Can you work these out from the model? Positions are in its coordinate system, mm. A direction names the side the tool comes from. Round coordinates to 2 decimals unless told otherwise and drop trailing zeros. Loops run counter-clockwise (first coordinate to the right, second up) from the corner with the lowest first, then second, coordinate; pieces in that order, holes last. Notation, with made-up numbers: M -2.75,17.5 L 28.25,17.5 A18 cw 28.25,42.5 Z; hole C 49.5,-19.5 d10. An arc over 180 degrees is marked long. Return JSON: item names as keys, results as strings.
```python
from build123d import *

# Parameters (mm, degrees)
SKETCH1_W           = 150
SKETCH1_H           = 150
BOSS_EXTRUDE1_DEPTH = 3
CUT_EXTRUDE1_DEPTH  = 264.0332057
SKETCH4_R           = 2.5
CUT_EXTRUDE2_DEPTH  = 3
SKETCH5_R           = 2
CUT_EXTRUDE3_DEPTH  = 10


with BuildPart() as part:
    # Sketch1 → Boss-Extrude1 (new body)
    with BuildSketch(Plane.XY):
        with Locations((146.896551724, 66.206896552)):
            Rectangle(SKETCH1_W, SKETCH1_H)
    extrude(amount=BOSS_EXTRUDE1_DEPTH)

    # Sketch2 → Cut-Extrude1 (cut, through all)
    with BuildSketch(Plane.XY.offset(3)):
        with BuildLine():
            ThreePointArc((188.163122783, 113.13032186), (146.896551724, 128.694797217), (105.629980666, 113.13032186))
            Line((105.629980666, 113.13032186), (112.718359737, 106.041942789))
            ThreePointArc((112.718359737, 106.041942789), (146.896551724, 118.694797217), (181.074743712, 106.041942789))
            Line((181.074743712, 106.041942789), (188.163122783, 113.13032186))
        make_face()
        with BuildLine():
            Line((107.061505487, 100.385088539), (99.973126416, 107.47346761))
            ThreePointArc((99.973126416, 107.47346761), (84.408651059, 66.206896552), (99.973126416, 24.940325493))
            Line((99.973126416, 24.940325493), (107.061505487, 32.028704564))
            ThreePointArc((107.061505487, 32.028704564), (94.408651059, 66.206896552), (107.061505487, 100.385088539))
        make_face()
        with BuildLine():
            ThreePointArc((209.384452389, 66.206896552), (205.363995952, 88.259009716), (193.819977032, 107.47346761))
            Line((193.819977032, 107.47346761), (186.731597961, 100.385088539))
            ThreePointArc((186.731597961, 100.385088539), (196.119705149, 84.429434333), (199.384452389, 66.206896552))
            ThreePointArc((199.384452389, 66.206896552), (196.119705149, 47.984358771), (186.731597961, 32.028704564))
            Line((186.731597961, 32.028704564), (193.819977032, 24.940325493))
            ThreePointArc((193.819977032, 24.940325493), (205.363995952, 44.154783387), (209.384452389, 66.206896552))
        make_face()
        with BuildLine():
            Line((112.718359737, 26.371850315), (105.629980666, 19.283471244))
            ThreePointArc((105.629980666, 19.283471244), (146.896551724, 3.718995886), (188.163122783, 19.283471244))
            Line((188.163122783, 19.283471244), (181.074743712, 26.371850315))
            ThreePointArc((181.074743712, 26.371850315), (146.896551724, 13.718995886), (112.718359737, 26.371850315))
        make_face()
        with BuildLine():
            ThreePointArc((150.896551724, 23.907703853), (176.940034403, 36.163413873), (189.195744423, 62.206896552))
            Line((189.195744423, 62.206896552), (179.137266506, 62.206896552))
            ThreePointArc((179.137266506, 62.206896552), (169.868966591, 43.234481685), (150.896551724, 33.96618177))
            Line((150.896551724, 33.96618177), (150.896551724, 23.907703853))
        make_face()
        with BuildLine():
            Line((114.655836942, 62.206896552), (104.597359026, 62.206896552))
            ThreePointArc((104.597359026, 62.206896552), (116.853069045, 36.163413873), (142.896551724, 23.907703853))
            Line((142.896551724, 23.907703853), (142.896551724, 33.96618177))
            ThreePointArc((142.896551724, 33.96618177), (123.924136857, 43.234481685), (114.655836942, 62.206896552))
        make_face()
        with BuildLine():
            Line((142.896551724, 98.447611333), (142.896551724, 108.50608925))
            ThreePointArc((142.896551724, 108.50608925), (116.853069045, 96.250379231), (104.597359026, 70.206896552))
            Line((104.597359026, 70.206896552), (114.655836942, 70.206896552))
            ThreePointArc((114.655836942, 70.206896552), (123.924136857, 89.179311419), (142.896551724, 98.447611333))
        make_face()
        with BuildLine():
            ThreePointArc((189.195744423, 70.206896552), (176.940034403, 96.250379231), (150.896551724, 108.50608925))
            Line((150.896551724, 108.50608925), (150.896551724, 98.447611333))
            ThreePointArc((150.896551724, 98.447611333), (169.868966591, 89.179311419), (179.137266506, 70.206896552))
            Line((179.137266506, 70.206896552), (189.195744423, 70.206896552))
        make_face()
        with BuildLine():
            Line((165.372753073, 79.026243651), (158.090015102, 71.74350568))
            ThreePointArc((158.090015102, 71.74350568), (159.056537781, 69.049853135), (159.384452389, 66.206896552))
            ThreePointArc((159.384452389, 66.206896552), (159.166880972, 63.885973637), (158.521748029, 61.645923641))
            Line((158.521748029, 61.645923641), (165.932760465, 54.234911206))
            ThreePointArc((165.932760465, 54.234911206), (168.504305512, 59.977076926), (169.384452389, 66.206896552))
            ThreePointArc((169.384452389, 66.206896552), (168.358106385, 72.923096956), (165.372753073, 79.026243651))
        make_face()
        with BuildLine():
            Line((134.077204625, 84.6830979), (141.359942596, 77.400359929))
            ThreePointArc((141.359942596, 77.400359929), (146.896551724, 78.694797217), (152.433160852, 77.400359929))
            Line((152.433160852, 77.400359929), (159.715898823, 84.6830979))
            ThreePointArc((159.715898823, 84.6830979), (146.896551724, 88.694797217), (134.077204625, 84.6830979))
        make_face()
        with BuildLine():
            ThreePointArc((135.703088346, 60.670287424), (134.408651059, 66.206896552), (135.703088346, 71.74350568))
            Line((135.703088346, 71.74350568), (128.420350375, 79.026243651))
            ThreePointArc((128.420350375, 79.026243651), (124.408651059, 66.206896552), (128.420350375, 53.387549452))
            Line((128.420350375, 53.387549452), (135.703088346, 60.670287424))
        make_face()
        with BuildLine():
            ThreePointArc((152.433160852, 55.013433174), (146.896551724, 53.718995886), (141.359942596, 55.013433174))
            Line((141.359942596, 55.013433174), (134.077204625, 47.730695203))
            ThreePointArc((134.077204625, 47.730695203), (146.896551724, 43.718995886), (159.715898823, 47.730695203))
            Line((159.715898823, 47.730695203), (152.433160852, 55.013433174))
        make_face()
    extrude(amount=-CUT_EXTRUDE1_DEPTH, mode=Mode.SUBTRACT)

    # Sketch4 → Cut-Extrude2 (cut)
    with BuildSketch(Plane.XY.offset(3)):
        with Locations((81.896551724, 131.206896552)):
            Circle(SKETCH4_R)
        with Locations((211.896551724, 131.206896552)):
            Circle(SKETCH4_R)
        with Locations((211.896551724, 1.206896552)):
            Circle(SKETCH4_R)
        with Locations((81.896551724, 1.206896552)):
            Circle(SKETCH4_R)
    extrude(amount=-CUT_EXTRUDE2_DEPTH, mode=Mode.SUBTRACT)

    # Sketch5 → Cut-Extrude3 (cut)
    with BuildSketch(Plane.XY.offset(3)):
        with Locations((146.896551724, 66.206896552)):
            Circle(SKETCH5_R)
    extrude(amount=-CUT_EXTRUDE3_DEPTH, mode=Mode.SUBTRACT)


solid = part.part
```
Q1. Suppose I cut it at C-C, the plane x = 176.5. Please give me the cut outline in (y, z).
Results:
{"outline": "M -8.79,0 L 11.18,0 L 11.18,3 L -8.79,3 Z; M 22.86,0 L 35.73,0 L 35.73,3 L 22.86,3 Z; M 52.82,0 L 79.59,0 L 79.59,3 L 52.82,3 Z; M 96.68,0 L 109.55,0 L 109.55,3 L 96.68,3 Z; M 121.24,0 L 141.21,0 L 141.21,3 L 121.24,3 Z"}
Q2. Suppose I cut it at A-A, the plane x = 87.5. Please give me the cut outline in (y, z), plus the area to 3 significant figures.
Results:
{"outline": "M -8.79,0 L 46.8,0 L 46.8,3 L -8.79,3 Z; M 85.62,0 L 141.21,0 L 141.21,3 L 85.62,3 Z", "area": "334 mm2"}
Q3. Suppose I cut it at D-D, the plane x = 207. Please give me the cut outline in (y, z).
Results:
{"outline": "M -8.79,0 L 49.11,0 L 49.11,3 L -8.79,3 Z; M 83.3,0 L 141.21,0 L 141.21,3 L 83.3,3 Z"}
Q4. On a 3-axis mill with a long thin cutter (end or side, diameter ignored), from which of +Z, -Z, +X, -X, +Y, -Y can I reach the whole of each face in a straight line? I mean faces 1 (the flat face through (184.669, 22.778, 1.521)), 2 (the flat face through (163, 51, 3)). Say none if no direction works.
Results:
{"face 1": "+Z, -Z", "face 2": "+Z, +X, -X, +Y, -Y"}
Q5. Suppose I cut it at B-B, the plane y = 36. Please give me the cut outline in (x, z).
Results:
{"outline": "M 71.9,0 L 92.19,0 L 92.19,3 L 71.9,3 Z; M 103.97,0 L 117.02,0 L 117.02,3 L 103.97,3 Z; M 134.94,0 L 158.86,0 L 158.86,3 L 134.94,3 Z; M 176.78,0 L 189.82,0 L 189.82,3 L 176.78,3 Z; M 201.6,0 L 221.9,0 L 221.9,3 L 201.6,3 Z"}
Q6. Thinking about a two-plate mould opening in X: for faces 3 (the flat face through (163, 51, 0)), 4 (the cylindrical face through (169.655, 89.391, 1.521)), 5 (the cylindrical face through (123.712, 88.965, 1.521)), which applies, pulls with the +X half, pulls with the -X half, needs draft (parallel to the pull), parting line crosses it, or undercut?
Results:
{"face 3": "needs draft", "face 4": "undercut", "face 5": "undercut"}
Q7. If I drill on line 1 along X through (y, z) = (99.5, 2.1); line 2 along X through (y, z) = (50, 2.2); line 3 along Y through (x, z) = (164, 0.6), over which ranges is the centre line in solid material (lowest first)?
Results:
{"line 1": "x = 71.9 to 94.02, 106.32 to 120.5, 142.9 to 150.9, 173.29 to 187.47, 199.78 to 221.9", "line 2": "x = 71.9 to 86.55, 96.97 to 107.62, 118.74 to 136.35, 157.45 to 175.05, 186.17 to 196.82, 207.25 to 221.9", "line 3": "y = -8.79 to 6.11, 16.58 to 27.31, 38.59 to 56.17, 77.65 to 93.83, 105.1 to 115.83, 126.31 to 141.21"}
